from build123d import *

# Parameters (mm, degrees)
SKETCH1_W           = 1.5
SKETCH1_H           = 9.05
SKETCH1_H_2         = 1.5
BOSS_EXTRUDE1_DEPTH = 1.5
SKETCH1_3_W         = 1.5
SKETCH1_3_H         = 1.5
BOSS_EXTRUDE2_DEPTH = 6
BOSS_EXTRUDE3_DEPTH = 1.5


with BuildPart() as part:
    # Sketch1 → Boss-Extrude1 (new body)
    with BuildSketch(Plane.XY):
        with Locations((0.75, 4.525)):
            Rectangle(SKETCH1_W, SKETCH1_H)
        with Locations((0.75, 9.8)):
            Rectangle(SKETCH1_W, SKETCH1_H_2)
        with Locations((0.75, -0.75)):
            Rectangle(SKETCH1_W, SKETCH1_H_2)
    extrude(amount=BOSS_EXTRUDE1_DEPTH)

    # Sketch1<3> → Boss-Extrude2 (add)
    with BuildSketch(Plane.XY):
        with Locations((0.75, 9.8)):
            Rectangle(SKETCH1_3_W, SKETCH1_3_H)
        with Locations((0.75, -0.75)):
            Rectangle(SKETCH1_3_W, SKETCH1_3_H)
    extrude(amount=-BOSS_EXTRUDE2_DEPTH)

    # Sketch2 → Boss-Extrude3 (add)
    with BuildSketch(Plane(origin=(1.5, 0, 0), x_dir=(0, 0, -1), z_dir=(1, 0, 0))):
        Polygon((4.5, 9.05), (6, 7.55), (6, 9.05), align=None)
        Polygon((6, 0), (4.5, 0), (6, 1.5), align=None)
    extrude(amount=-BOSS_EXTRUDE3_DEPTH)


solid = part.part
Input: part model. Units: mm. Frame: model coordinates. A direction names the side the tool comes from. Round coordinates to 2 decimals unless told otherwise and drop trailing zeros. Write each loop counter-clockwise with the first axis right and the second up, starting at its lowest first coordinate (ties: lowest second). Pieces come first, ordered by that corner, then holes.
1) Reachability of faces 1 (the flat face through (1, 5, 0)), 2 (the flat face through (1, 5, 1.5)) from +Z, -Z, +X, -X, +Y, -Y: full face, straight path, thin tool, end or side. Return the list, or none.
2) Ray query, L1, parallel to Y at x = 0.4, z = -1.75; L2, parallel to Z at x = 0.1, y = 3; L3, parallel to Z at x = 0.35, y = 9. Return the intervals inside material, ascending.
3) Cut plane C-C (x = 1.25). Return the cut outline in (y, z), then the cut area to 3 significant figures.
4) Cut plane D-D (y = 2.75). Return the cut outline in (x, z).
5) Cut plane B-B (z = -5). Return the cut outline in (x, y), then the cut area to 3 significant figures.
6) Draft query along Z for faces 3 (the flat face through (0, 4.6, 0.3)), 4 (the flat face through (1, 0, -6)), 5 (the flat face through (1, 0, -2)), 6 (the flat face through (0.8, 0.7, -5.2)). Return one class per face: pulls with the +Z half, pulls with the -Z half, needs draft (parallel to the pull), parting line crosses it, or undercut.
7) Cut plane A-A (y = 8.75). Return the cut outline in (x, z).
Geometry says:
1. face 1: +X, -X
1. face 2: +Z, +X, -X, +Y, -Y
2. L1: y = -1.5 to 0, 9.05 to 10.55
2. L2: z = 0 to 1.5
2. L3: z = -6 to -4.55, 0 to 1.5
3. outline: (-1.5, -6) - (1.5, -6) - (0, -4.5) - (0, 0) - (9.05, 0) - (9.05, -4.5) - (7.55, -6) - (10.55, -6) - (10.55, 1.5) - (-1.5, 1.5) - close
3. area: 38.3 mm2
4. outline: (0, 0) - (1.5, 0) - (1.5, 1.5) - (0, 1.5) - close
5. outline: (0, -1.5) - (1.5, -1.5) - (1.5, 0.5) - (0, 0.5) - close; (0, 8.55) - (1.5, 8.55) - (1.5, 10.55) - (0, 10.55) - close
5. area: 6.00 mm2
6. face 3: needs draft
6. face 4: pulls with the -Z half
6. face 5: undercut
6. face 6: undercut
7. outline: (0, -6) - (1.5, -6) - (1.5, -4.8) - (0, -4.8) - close; (0, 0) - (1.5, 0) - (1.5, 1.5) - (0, 1.5) - close
